from build123d import *

# Parameters (mm, degrees)
F0_R     = 12
F1_DEPTH = 3
F2_DEPTH = 23
F4_START = 18
F4_DEPTH = 5
F5_SIZE  = 3
F6_W     = 15.1
F6_H     = 20
F7_DEPTH = 52.8


with BuildPart() as f1:
    # F0 (on Top) → F1 (new body)
    with BuildSketch(Plane.XY):
        with BuildLine():
            ThreePointArc((0, -50), (35.3553390593, -35.3553390593), (50, 0))
            ThreePointArc((50, 0), (-35.3553390593, 35.3553390593), (0, -50))
        make_face()
        Circle(F0_R, mode=Mode.SUBTRACT)
    extrude(amount=F1_DEPTH)

    # F0 (on Top) → F2 (join)
    with BuildSketch(Plane.XY):
        with BuildLine():
            ThreePointArc((52.5, 0), (-37.1231060123, 37.1231060123), (0, -52.5))
            ThreePointArc((0, -52.5), (37.1231060123, -37.1231060123), (52.5, 0))
        make_face()
        with BuildLine():
            ThreePointArc((0, -50), (-35.3553390593, 35.3553390593), (50, 0))
            ThreePointArc((50, 0), (35.3553390593, -35.3553390593), (0, -50))
        make_face(mode=Mode.SUBTRACT)
    extrude(amount=F2_DEPTH)

    # F3 (on Top) → F4 (join)
    with BuildSketch(Plane.XY.offset(F4_START)):
        with BuildLine():
            Line((31.8198051534, -31.8198051534), (35.3553390593, -35.3553390593))
            ThreePointArc((35.3553390593, -35.3553390593), (46.1939766256, -19.1341716183), (50, 0))
            Line((50, 0), (45, 0))
            ThreePointArc((45, 0), (41.574578963, -17.2207544564), (31.8198051534, -31.8198051534))
        make_face()
        with BuildLine():
            ThreePointArc((-45, 0), (-41.574578963, 17.2207544564), (-31.8198051534, 31.8198051534))
            Line((-31.8198051534, 31.8198051534), (-35.3553390593, 35.3553390593))
            ThreePointArc((-35.3553390593, 35.3553390593), (-46.1939766256, 19.1341716183), (-50, 0))
            Line((-50, 0), (-45, 0))
        make_face()
        with BuildLine():
            ThreePointArc((35.3553390593, 35.3553390593), (19.1341716183, 46.1939766256), (0, 50))
            Line((0, 50), (0, 45))
            ThreePointArc((0, 45), (17.2207544564, 41.574578963), (31.8198051534, 31.8198051534))
            Line((31.8198051534, 31.8198051534), (35.3553390593, 35.3553390593))
        make_face()
        with BuildLine():
            Line((-31.8198051534, -31.8198051534), (-35.3553390593, -35.3553390593))
            ThreePointArc((-35.3553390593, -35.3553390593), (-19.1341716183, -46.1939766256), (0, -50))
            Line((0, -50), (0, -45))
            ThreePointArc((0, -45), (-17.2207544564, -41.574578963), (-31.8198051534, -31.8198051534))
        make_face()
    extrude(amount=F4_DEPTH)

    # F5
    f5_edges = [f1.edges().sort_by_distance(p)[0] for p in [
        (0, 52.5, 0),
    ]]
    chamfer(f5_edges, length=F5_SIZE)

    # F6 (on face) → F7 (cut)
    with BuildSketch(Plane.XY.offset(3)):
        with Locations((0, 37.4)):
            Rectangle(F6_W, F6_H)
    extrude(amount=-F7_DEPTH, mode=Mode.SUBTRACT)


solid = f1.part
Source: CAD feature listing. Evaluate the final solid. Frame: model axes, mm. A direction names the side the tool comes from. Give positions to 0.01 mm unless a question says otherwise; leave off trailing zeros. Order: outer loops, then holes, each group sorted by start corner. A loop starts at its lowest first (then second) coordinate and runs counter-clockwise, first axis right, second up. Notation, with made-up numbers: (74.25, 52) -> (133.25, 52) arc R18 ccw to (133.25, 69) -> close; hole circle Ø8 at (-20.75, 51). An arc over 180 degrees is marked (long way). Write item = value, one per line.
Q1. Material intervals for line 1 (Y direction, x = -28, z = 10); line 2 (Y direction, x = -2, z = 11.75); line 3 (Z direction, x = 38, y = -6), sorted ascending. Write a range as from..to.
Data:
line_1 = -44.41..-41.42, 41.42..44.41
line_2 = -52.46..-49.96, 49.96..52.46
line_3 = 0..3
Q2. Set-up query: faces 1 (the face through (-18, -42, 18)), 2 (the face through (-7.55, 37, 2)), 3 (the face through (-16.99, -41.67, 20.46)). Return all of +Z, -Z, +X, -X, +Y, -Y with unobstructed straight access to the full face (end or side cutting, diameter ignored); none if empty.
Data:
face_1 = none
face_2 = +Z, -Z
face_3 = +Z
Q3. Cut plane B-B, the plane z = 6. Output: boundary loops of the cut face in (x, y).
Data:
outline = circle Ø105 at (0, 0); hole circle Ø100 at (0, 0)
Q4. Pull-direction query (X, two-part tool) for faces 4 (the face through (0, 27.4, 2)), 5 (the face through (7.55, 37, 2)), 6 (the face through (10, -10, 0)), 7 (the face through (-30.21, 39.4, 0.15)); classes: released by +X, released by -X, zero draft, split by the parting line, or undercut.
Data:
face_4 = undercut
face_5 = undercut
face_6 = zero draft
face_7 = split by the parting line
Q5. Cut plane A-A, the plane z = 19.75. Output: boundary loops of the cut face in (x, y), and give its area (3 significant figures).
Data:
outline = circle Ø105 at (0, 0); hole (-50, 0) arc R50 ccw to (-35.36, -35.36) -> (-31.82, -31.82) arc R45 ccw to (0, -45) -> (0, -50) arc R50 ccw to (35.36, -35.36) -> (31.82, -31.82) arc R45 ccw to (45, 0) -> (50, 0) arc R50 ccw to (35.36, 35.36) -> (31.82, 31.82) arc R45 ccw to (0, 45) -> (0, 50) arc R50 ccw to (-35.36, 35.36) -> (-31.82, 31.82) arc R45 ccw to (-45, 0) -> close
area = 1,550 mm^2
Q6. Pin query (flat end, axial travel): pin 1 (3.5 mm diameter, centred on x = 3, z = 1, fed in from +Y); pin 2 (10 mm diameter, centred on x = -10.5, y = 34, fed in from +Z); pin 3 (1.5 mm diameter, centred on y = 41.5, z = 1.5, fed in from -X); pin 4 (14.5 mm diameter, centred on x = 44, y = -13, fed in from -Z). Return the tip coordinate at first contact, or that it passes through.
Data:
pin_1 = 52.17
pin_2 = 3
pin_3 = -31.26
pin_4 = 0
